from build123d import *

# Parameters (mm, degrees)
F0_W         = 25.4
F0_H         = 25.4
F1_DEPTH     = 25.4
F2_W         = 5.424141106
F2_H         = 6.936683166
F2_W_2       = 5.0867797479
F2_H_2       = 3.4590791911
F3_DEPTH     = 2.54
F4_R         = 1.9260545118
F4_R_2       = 1.1454537096
F5_DEPTH     = 2.54
F7_DEPTH     = 2.54
F8_W         = 27.94
F8_H         = 9.2223960251
F9_DEPTH     = 2.54
F10_W        = 27.94
F10_H        = 12.7
F11_DEPTH    = 2.54
F12_T1_DEPTH = 15.6041495789
F12_T6_DEPTH = 15.6041495789
F13_W        = 4.5640636235
F13_H        = 25.4
F14_DEPTH    = 5.08
F15_T1_DEPTH = 38.4641495789
F16_R        = 5.08
F17_R        = 2.413
F18_DEPTH    = 10.16


# Not quite as in the source:
# - a fillet or chamfer that OpenCascade refuses, or shapes differently, is made with other operations: its cross-section is extruded or revolved along the edge and cut away or added


with BuildPart() as f1:
    # F0 (on Top) → F1 (new body)
    with BuildSketch(Plane.XY):
        Rectangle(F0_W, F0_H)
    extrude(amount=-F1_DEPTH)

    # F2 (on face) → F3 (join)
    with BuildSketch(Plane.XZ.offset(12.7)):
        Polygon((-12.7, -19.636683166), (-12.7, -25.4), (12.7, -25.4), (12.7, -19.636683166), (7.6132202521, -19.636683166), (-7.275858894, -19.636683166), align=None)
        with Locations((-9.987929447, -16.168341583)):
            Rectangle(F2_W, F2_H)
        with Locations((10.156610126, -17.9071435705)):
            Rectangle(F2_W_2, F2_H_2)
    extrude(amount=F3_DEPTH)

    # F4 (on face) → F5 (join)
    with BuildSketch(Plane.XZ.offset(12.7)):
        with Locations((-7.3823751882, -4.9585988745)):
            Circle(F4_R)
        with Locations((6.6054924391, -5.1089939661)):
            Circle(F4_R_2)
    extrude(amount=F5_DEPTH)

    # F6 (on face) → F7 (join)
    with BuildSketch(Plane.XZ.offset(12.7)):
        Polygon((3.2856935422, -9.4954269007), (-3.2856935422, -9.4954269007), (0, -15.1864150539), align=None)
    extrude(amount=F7_DEPTH)

    # F8 (on face) → F9 (join)
    with BuildSketch(Plane.YZ.offset(12.7)):
        with Locations((-1.27, -20.7888019875)):
            Rectangle(F8_W, F8_H)
    extrude(amount=F9_DEPTH)

    # F10 (on face) → F11 (join)
    with BuildSketch(Plane(origin=(-12.7, 0, 0), x_dir=(0, -1, 0), z_dir=(-1, 0, 0))):
        with Locations((1.27, -19.05)):
            Rectangle(F10_W, F10_H)
    extrude(amount=F11_DEPTH)

    # F12: chamfer of 5.08 on 2 edges, made by hand

    # F12_s2 → F12_t1 (cut)
    with BuildSketch(Plane.XZ.offset(12.7)):
        Polygon((-7.275858894, -17.78), (-12.355858894, -12.7), (-7.275858894, -12.7), align=None)
    extrude(amount=F12_T1_DEPTH, mode=Mode.SUBTRACT)


with BuildPart() as f12_tool4:
    # F12_s5 → F12_t6 (new body)
    with BuildSketch(Plane.XZ.offset(12.7)):
        Polygon((7.6132202521, -21.2576039749), (12.6932202521, -16.1776039749), (7.6132202521, -16.1776039749), align=None)
    extrude(amount=F12_T6_DEPTH)

    split(bisect_by=Plane.XY.offset(-19.636683166), keep=Keep.TOP)


with BuildPart() as f1_1:
    add(f1.part)

    # F12_t3: cut F12_tool4
    add(f12_tool4.part, mode=Mode.SUBTRACT)

    # F13 (on face) → F14 (join)
    with BuildSketch(Plane.XY):
        with Locations((0.04063081, 0)):
            Rectangle(F13_W, F13_H)
    extrude(amount=F14_DEPTH)

    # F15: chamfer of 2.54 on 2 edges, made by hand

    # F15_s2 → F15_t1 (cut)
    with BuildSketch(Plane.XZ.offset(-19.2320747894)):
        Polygon((2.3226626217, 2.54), (-0.2173373783, 5.08), (2.3226626217, 5.08), align=None)
        Polygon((-2.2414010018, 2.54), (0.2985989982, 5.08), (-2.2414010018, 5.08), align=None)
    extrude(amount=F15_T1_DEPTH, mode=Mode.SUBTRACT)

    # F16
    f16_edges = [f1_1.edges().sort_by_distance(p)[0] for p in [
        (15.24, -1.27, -25.4),
        (-15.24, -1.27, -25.4),
    ]]
    fillet(f16_edges, radius=F16_R)

    # F17 (on face) → F18 (join)
    with BuildSketch(Plane(origin=(0, 0, -25.4), x_dir=(1, 0, 0), z_dir=(0, 0, -1))):
        Circle(F17_R)
    extrude(amount=F18_DEPTH)


solid = f1_1.part
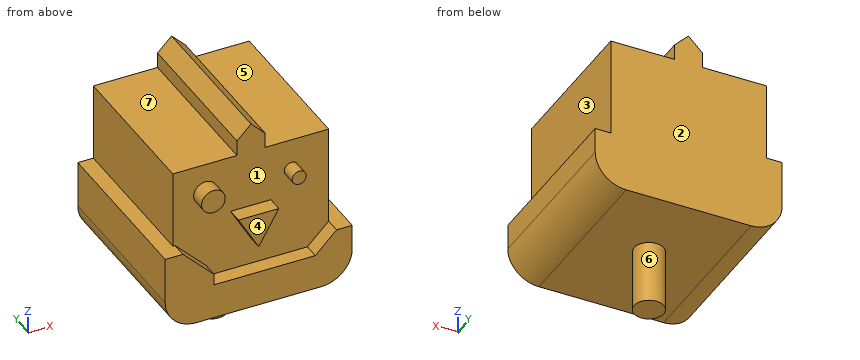
The model under review builds one solid part; all positions refer to its coordinate system, in mm. Face numbers are marked on the shaded views. A direction names the side the tool comes from. Give positions to 0.01 mm unless a question says otherwise; leave off trailing zeros. Order: outer loops, then holes, each group sorted by start corner. A loop starts at its lowest first (then second) coordinate and runs counter-clockwise, first axis right, second up. Notation, with made-up numbers: M -37,-22.5 L -4,-22.5 A17 cw -4,-4.5 Z; hole C 87.25,38 d7. An arc over 180 degrees is marked long. Use one line per item in the form item = value. Start each with the question number.
Item 1: Insertion check: pin 1 Ø3 at (x, y) = (-1.5, -14) entering from +Z; pin 2 Ø12 at (x, z) = (3.5, -2.5) entering from -Y; pin 3 Ø1 at (x, z) = (3.5, -29.5) entering from -Y; pin 4 Ø1.3 at (y, z) = (2.5, 1) entering from +X. Each pin has a flat end and moves straight along its axis. Give the tip position at first contact, or say it passes through.
Item 2: We need section D-D on y = -7.25. Give the boundary of the cut face in (x, z).
Item 3: We need section B-B on z = -7.5. Give the boundary of the cut face in (x, y), plus the area to 3 significant figures.
Item 4: The part is to be moulded in two halves that separate along X. For the marked faces 1, 2 and 3, say which applies: pulls with the +X half, pulls with the -X half, needs draft (parallel to the pull), parting line crosses it, or undercut.
Item 5: For the marked faces 4, 5, 6 and 7, list the 3-axis set-ups (+Z, -Z, +X, -X, +Y, -Y) from which the entire face can be reached by the end or side of a thin tool; tool diameter is ignored.
Item 6: We need section C-C on x = 7. Give the boundary of the cut face in (y, z).
Item 7: We need section A-A on y = 0. Give the boundary of the cut face in (x, z).
Item 8: To check wall thickness, follow line 1 along Y through (x, z) = (-1, -6.5); line 2 along Z through (x, y) = (-4.5, 6). State the ranges of each line that lie inside material, in increasing order. Write a range as from..to.
Completed:
q1.pin_1 = 4.03
q1.pin_2 = -15.24
q1.pin_3 = through
q1.pin_4 = 2.32
q2.outline = M -15.24,-20.32 A5.08 ccw -10.16,-25.4 L 10.16,-25.4 A5.08 ccw 15.24,-20.32 L 15.24,-16.18 L 12.7,-16.18 L 12.7,0 L 2.32,0 L 2.32,2.54 L 0.04,4.82 L -2.24,2.54 L -2.24,0 L -12.7,0 L -12.7,-12.7 L -15.24,-12.7 Z
q3.outline = M -12.7,-12.7 L 12.7,-12.7 L 12.7,12.7 L -12.7,12.7 Z
q3.area = 645 mm²
q4.face_1 = undercut
q4.face_2 = needs draft
q4.face_3 = pulls with the +X half
q5.face_4 = +Z, -Z, +X, -X, -Y
q5.face_5 = +Z, +X, +Y, -Y
q5.face_6 = -Z
q5.face_7 = +Z, -X, +Y, -Y
q6.outline = M -15.24,-25.4 L 12.7,-25.4 L 12.7,0 L -12.7,0 L -12.7,-4.03 L -15.24,-4.03 L -15.24,-6.18 L -12.7,-6.18 L -12.7,-19.64 L -15.24,-19.64 Z
q7.outline = M -15.24,-20.32 A5.08 ccw -10.16,-25.4 L -2.41,-25.4 L -2.41,-35.56 L 2.41,-35.56 L 2.41,-25.4 L 10.16,-25.4 A5.08 ccw 15.24,-20.32 L 15.24,-16.18 L 12.7,-16.18 L 12.7,0 L 2.32,0 L 2.32,2.54 L 0.04,4.82 L -2.24,2.54 L -2.24,0 L -12.7,0 L -12.7,-12.7 L -15.24,-12.7 Z
q8.line_1 = -12.7..12.7
q8.line_2 = -25.4..0
